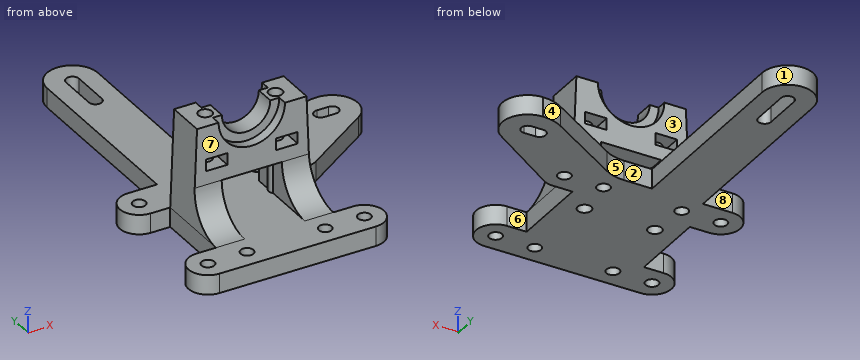
from build123d import *

# Parameters (mm, degrees)
RESSALTO_EXTRUS_O1_DEPTH = 5
ESBO_O2_W                = 5.5
ESBO_O2_H                = 3
RESSALTO_EXTRUS_O2_DEPTH = 10
ESBO_O4_W                = 8.5
ESBO_O4_H                = 2.5
ESBO_O6_R                = 1.75
CORTE_EXTRUS_O2_DEPTH    = 92.337287019
ESBO_O7_R                = 1.65
CORTE_EXTRUS_O3_DEPTH    = 10
ESBO_O8_R                = 1.65
RESSALTO_EXTRUS_O3_DEPTH = 5
FILETE3_R                = 10
FILETE4_R                = 10


with BuildPart() as part:
    # Esboço1 → Ressalto-extrusão1 (new body)
    with BuildSketch(Plane.XY):
        with BuildLine():
            Line((0.5, 68), (0.5, 33.5))
            Line((0.5, 33.5), (0.5, 20))
            Line((0.5, 20), (10.5, 20))
            Line((10.5, 20), (34, 34.5))
            Line((34, 34.5), (37, 34.5))
            ThreePointArc((37, 34.5), (43.5, 28), (37, 21.5))
            Line((37, 21.5), (15, 21.5))
            Line((15, 21.5), (15, -20))
            Line((15, -20), (-15, -20))
            Line((-15, -20), (-15, 20))
            Line((-15, 20), (-12.5, 20))
            Line((-12.5, 20), (-12.5, 68))
            ThreePointArc((-12.5, 68), (-6, 74.5), (0.5, 68))
        make_face()
        with BuildLine():
            Line((-4.35, 68), (-4.35, 58))
            ThreePointArc((-4.35, 58), (-6, 56.35), (-7.65, 58))
            Line((-7.65, 58), (-7.65, 68))
            ThreePointArc((-7.65, 68), (-6, 69.65), (-4.35, 68))
        make_face(mode=Mode.SUBTRACT)
        with BuildLine():
            Line((34, 26.35), (37, 26.35))
            ThreePointArc((37, 26.35), (38.65, 28), (37, 29.65))
            Line((37, 29.65), (34, 29.65))
            ThreePointArc((34, 29.65), (32.35, 28), (34, 26.35))
        make_face(mode=Mode.SUBTRACT)
    extrude(amount=RESSALTO_EXTRUS_O1_DEPTH)

    # Esboço2 → Ressalto-extrusão2 (add)
    with BuildSketch(Plane(origin=(0, 0, 0), x_dir=(1, 0, 0), z_dir=(0, 1, 0))):
        with BuildLine():
            Line((14, -30), (15, -5))
            Line((15, -5), (7.7, -5))
            Line((7.7, -5), (7.7, -15))
            Line((7.7, -15), (-7.7, -15))
            Line((-7.7, -15), (-7.7, -5))
            Line((-7.7, -5), (-15, -5))
            Line((-15, -5), (-14, -30))
            Line((-14, -30), (-6.2, -30))
            ThreePointArc((-6.2, -30), (0, -23.8), (6.2, -30))
            Line((6.2, -30), (14, -30))
        make_face()
        with Locations((-9, -20)):
            Rectangle(ESBO_O2_W, ESBO_O2_H, mode=Mode.SUBTRACT)
        with Locations((9, -20)):
            Rectangle(ESBO_O2_W, ESBO_O2_H, mode=Mode.SUBTRACT)
    extrude(amount=RESSALTO_EXTRUS_O2_DEPTH)

    # Esboço4 → Corte-Revolução3 (revolve, cut)
    with BuildSketch(Plane(origin=(0, 0, 0), x_dir=(0, 0, -1), z_dir=(1, 0, 0))):
        with Locations((-25.75, 8.75)):
            Rectangle(ESBO_O4_W, ESBO_O4_H)
        with Locations((-25.75, 1.25)):
            Rectangle(ESBO_O4_W, ESBO_O4_H)
    revolve(axis=Axis((0, 10, 30), (0, -1, 0)), mode=Mode.SUBTRACT)

    # Esboço6 → Corte-extrusão2 (cut, through all)
    with BuildSketch(Plane.XY.offset(30)):
        with Locations((-9, 5)):
            Circle(ESBO_O6_R)
        with Locations((9, 5)):
            Circle(ESBO_O6_R)
    extrude(amount=-CORTE_EXTRUS_O2_DEPTH, mode=Mode.SUBTRACT)

    # Esboço7 → Corte-extrusão3 (cut)
    with BuildSketch(Plane.XY.offset(5)):
        with Locations((-10, 15)):
            Circle(ESBO_O7_R)
        with Locations((-10, -15)):
            Circle(ESBO_O7_R)
        with Locations((10, -15)):
            Circle(ESBO_O7_R)
        with Locations((10, 15)):
            Circle(ESBO_O7_R)
    extrude(amount=-CORTE_EXTRUS_O3_DEPTH, mode=Mode.SUBTRACT)

    # Esboço8 → Ressalto-extrusão3 (add)
    # profile 1 of 4: a face of its own
    with BuildSketch(Plane(origin=(0, 0, 0), x_dir=(-1, 0, 0), z_dir=(0, 0, -1))):
        with BuildLine():
            Line((20, 20), (15, 20))
            Line((15, 20), (15, 10))
            Line((15, 10), (20, 10))
            ThreePointArc((20, 10), (25, 15), (20, 20))
        make_face()
        with Locations((20, 15)):
            Circle(ESBO_O8_R, mode=Mode.SUBTRACT)
    # profile 2 of 4: a face of its own
    with BuildSketch(Plane(origin=(0, 0, 0), x_dir=(-1, 0, 0), z_dir=(0, 0, -1))):
        with BuildLine():
            Line((-15, 10), (-20, 10))
            ThreePointArc((-20, 10), (-21.436224898, 10.210714245), (-22.751396578, 10.825096783))
            Line((-22.751396578, 10.825096783), (-40.576815551, 22.572625818))
            ThreePointArc((-40.576815551, 22.572625818), (-38.867092367, 21.773928519), (-37, 21.5))
            Line((-37, 21.5), (-15, 21.5))
            Line((-15, 21.5), (-15, 10))
        make_face()
        with Locations(Location((-20, 15, 0), (0, 0, 180))):
            Circle(ESBO_O8_R, mode=Mode.SUBTRACT)
    # profile 3 of 4: a face of its own
    with BuildSketch(Plane(origin=(0, 0, 0), x_dir=(-1, 0, 0), z_dir=(0, 0, -1))):
        with BuildLine():
            Line((15, -10), (20, -10))
            ThreePointArc((20, -10), (25, -15), (20, -20))
            Line((20, -20), (15, -20))
            Line((15, -20), (15, -10))
        make_face()
        with Locations(Location((20, -15, 0), (0, 0, 180))):
            Circle(ESBO_O8_R, mode=Mode.SUBTRACT)
    # profile 4 of 4: a face of its own
    with BuildSketch(Plane(origin=(0, 0, 0), x_dir=(-1, 0, 0), z_dir=(0, 0, -1))):
        with BuildLine():
            Line((-20, -20), (-15, -20))
            Line((-15, -20), (-15, -10))
            Line((-15, -10), (-20, -10))
            ThreePointArc((-20, -10), (-25, -15), (-20, -20))
        make_face()
        with Locations((-20, -15)):
            Circle(ESBO_O8_R, mode=Mode.SUBTRACT)
    extrude(amount=-RESSALTO_EXTRUS_O3_DEPTH)

    # Filete3
    filete3_edges = [part.edges().sort_by_distance(p)[0] for p in [
        (10.5, 20, 2.5),
        (34, 34.5, 2.5),
    ]]
    fillet(filete3_edges, radius=FILETE3_R)

    # Filete4
    filete4_edges = [part.edges().sort_by_distance(p)[0] for p in [
        (-11.35, 0, 5),
        (11.35, 0, 5),
    ]]
    fillet(filete4_edges, radius=FILETE4_R - 0.0001)  # a hair under: the kernel refuses the full size


solid = part.part
Model file for the job. Use its own axes, mm. Face numbers are marked on the shaded views. A direction names the side the tool comes from. Give positions to 0.01 mm unless a question says otherwise; leave off trailing zeros. Loops run counter-clockwise (first coordinate to the right, second up) from the corner with the lowest first, then second, coordinate; pieces in that order, holes last. Notation, with made-up numbers: (89.5, 20.25) -> (126.5, 20.25) arc R4 ccw to (126.5, 26.25) -> close; hole circle Ø9 at (73, 2). An arc over 180 degrees is marked (long way). Use a Markdown table: item, result. Add a question column.
(1) Drop flat-ended pins along their axis: pin 1 Ø4 at (x, z) = (-16.5, 3.5) entering from +Y; pin 2 Ø3 at (y, z) = (-3.5, 8) entering from +X; pin 3 Ø4 at (y, z) = (62, 3.5) entering from +X. Give the stop position or say it passes through.
(2) Slice it at B-B on z = 9. List the corners of the cut face in (x, y).
(3) Wall check: line 1 along Y through (x, z) = (-9, 25.25); line 2 along Z through (x, y) = (-9, 69); line 3 along X through (y, z) = (2, 6.5). Give the ranges that are in metal, low to high.
(4) Slice it at D-D on z = 2. Give the number of separate pieces and of enclosed holes in the cut face, and give its area (3 significant figures).
(5) Slice it at A-A on x = 4.5. List the corners of the cut face in (y, z), and give its area (3 significant figures).
(6) Tool access for the marked faces 5, 6, 7 and 8: list every direction of +Z, -Z, +X, -X, +Y, -Y with a clear straight run to the whole face (end or side of a thin tool).
(7) Slice it at C-C on y = 28. List the corners of the cut face in (x, z).
(8) Mould opens along X. For the marked faces 1, 2, 3 and 4 say: +X half, -X half, draft (parallel to the pull), parting line (faces both ways), or undercut.
Filled sheet:
| question | item | result |
|---|---|---|
| 1 | pin 1 | y = 20 |
| 1 | pin 2 | x = 14.94 |
| 1 | pin 3 | x = 0.5 |
| 2 | outline | (-14.84, -2) -> (-7.7, -2) -> (-7.7, 3.83) arc R1.75 cw (long way) to (-7.7, 6.17) -> (-7.7, 10) -> (-14.84, 10) -> close; (7.7, -2) -> (14.84, -2) -> (14.84, 10) -> (7.7, 10) -> (7.7, 6.17) arc R1.75 cw (long way) to (7.7, 3.83) -> close |
| 3 | line 1 | 0 to 3.25, 6.75 to 10 |
| 3 | line 2 | 0 to 5 |
| 3 | line 3 | -14.94 to -7.7, 7.7 to 14.94 |
| 4 | separate pieces | 1 |
| 4 | enclosed holes | 12 |
| 4 | area | 2,430 mm2 |
| 5 | outline | (-20, 0) -> (20, 0) -> (20, 5) -> (-20, 5) -> close; (0, 15) -> (10, 15) -> (10, 22.79) -> (7.5, 22.79) -> (7.5, 25.74) -> (2.5, 25.74) -> (2.5, 22.79) -> (0, 22.79) -> close |
| 5 | area | 293 mm2 |
| 6 | face 5 | +Z, -Z, +Y |
| 6 | face 6 | +Z, -Z, +X |
| 6 | face 7 | +Z, +X, -X, -Y |
| 6 | face 8 | +Z, -Z, -X, +Y |
| 7 | outline | (-12.5, 0) -> (0.5, 0) -> (0.5, 5) -> (-12.5, 5) -> close; (23.47, 0) -> (32.35, 0) -> (32.35, 5) -> (23.47, 5) -> close; (38.65, 0) -> (43.5, 0) -> (43.5, 5) -> (38.65, 5) -> close |
| 8 | face 1 | parting line |
| 8 | face 2 | undercut |
| 8 | face 3 | draft |
| 8 | face 4 | undercut |
